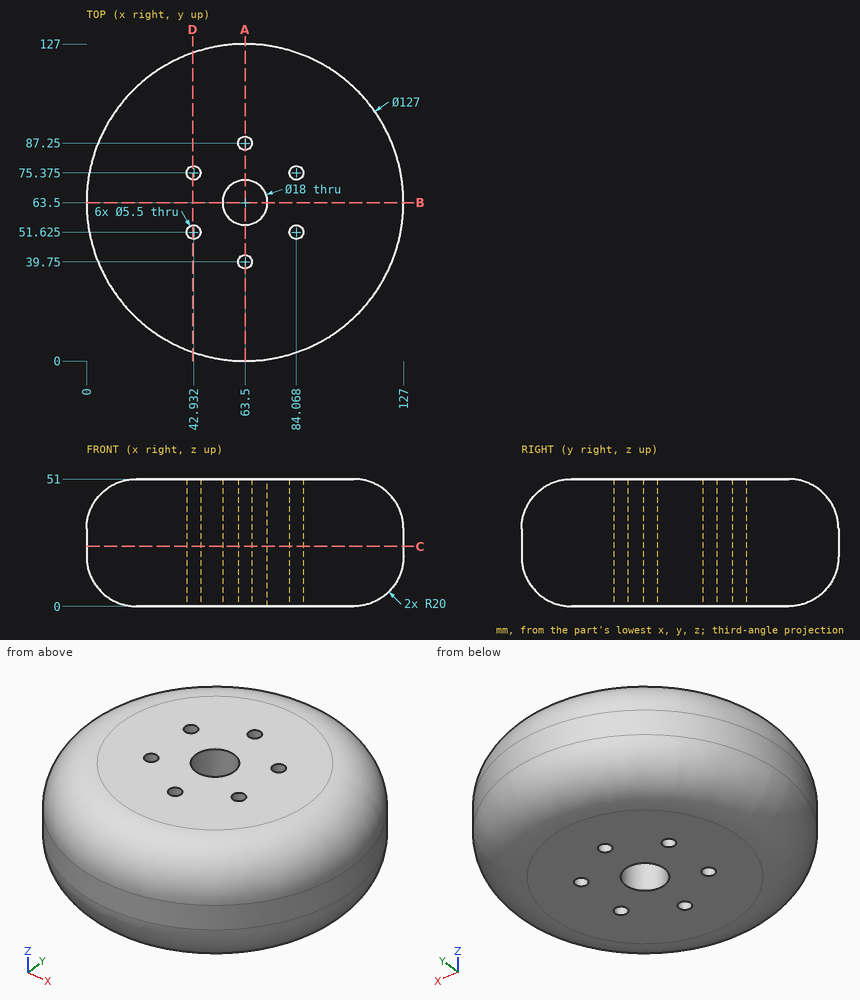
Study the drawing (mm; zero at the part's minimum x, y, z) and answer. Coordinates: 2 decimals unless noted, no trailing zeros. Loops run counter-clockwise (first coordinate to the right, second up) from the corner with the lowest first, then second, coordinate; pieces in that order, holes last. Notation, with made-up numbers: (5, 2) -> (60, 2) arc R17 cw to (60, 9) -> close; hole circle Ø1 at (-37, 26.5). An arc over 180 degrees is marked (long way). Write item = value, one per line. Start each with the question number.
1) The part is cut by section A-A, the plane x = 63.5. Determine the outline of the cut face in (y, z).
2) Find the intervals of material crossed by L1, parallel to Y at x = 63.5, z = 29; L2, parallel to Y at x = 63.5, z = 13 (3 decimals); L3, parallel to X at y = 53, z = 39, in increasing order. Write a range as from..to.
3) The part is cut by section D-D, the plane x = 42.5. State how many separate pieces and enclosed holes the cut face has, plus the area to 3 significant figures.
4) Given P1, Ø6, axis at x = 32, z = 11.5, coming from the -Y side; P2, Ø4, axis at y = 66.5, z = 24, coming from the +X side; P3, Ø1.5, axis at y = 39, z = 19, coming from the +X side; P4, Ø9, axis at x = 63.5, y = 87.25, coming from the -Z side, each flat-ended and moving along its own axis, determine where each tip first touches the part or whether it passes through.
5) The part is cut by section B-B, the plane y = 63.5. Determine the outline of the cut face in (x, z).
6) The part is cut by section C-C, the plane z = 24. Determine the outline of the cut face in (x, y) (3 decimals), plus the area to 3 significant figures.
Result:
q1.outline = (0, 20) arc R20 ccw to (20, 0) -> (37, 0) -> (37, 51) -> (20, 51) arc R20 ccw to (0, 31) -> close; (42.5, 0) -> (54.5, 0) -> (54.5, 51) -> (42.5, 51) -> close; (72.5, 0) -> (84.5, 0) -> (84.5, 51) -> (72.5, 51) -> close; (90, 0) -> (107, 0) arc R20 ccw to (127, 20) -> (127, 31) arc R20 ccw to (107, 51) -> (90, 51) -> close
q2.L1 = 0..37, 42.5..54.5, 72.5..84.5, 90..127
q2.L2 = 1.265..37, 42.5..54.5, 72.5..84.5, 90..125.735
q2.L3 = 2.57..40.55, 45.31..81.69, 86.45..124.43
q3.separate_pieces = 3
q3.enclosed_holes = 0
q3.area = 5,190 mm²
q4.P1 = 8.36
q4.P2 = 126.99
q4.P3 = 122.37
q4.P4 = 0
q5.outline = (0, 20) arc R20 ccw to (20, 0) -> (54.5, 0) -> (54.5, 51) -> (20, 51) arc R20 ccw to (0, 31) -> close; (72.5, 0) -> (107, 0) arc R20 ccw to (127, 20) -> (127, 31) arc R20 ccw to (107, 51) -> (72.5, 51) -> close
q6.outline = circle Ø127 at (63.5, 63.5); hole circle Ø5.5 at (42.932, 51.625); hole circle Ø5.5 at (42.932, 75.375); hole circle Ø18 at (63.5, 63.5); hole circle Ø5.5 at (63.5, 39.75); hole circle Ø5.5 at (63.5, 87.25); hole circle Ø5.5 at (84.068, 51.625); hole circle Ø5.5 at (84.068, 75.375)
q6.area = 12,300 mm²
